Source: three-view drawing plus pictorial views. Frame: mm from the lowest corner of the part. Give positions to 0.01 mm unless a question says otherwise; leave off trailing zeros. Loops run counter-clockwise (first coordinate to the right, second up) from the corner with the lowest first, then second, coordinate; pieces in that order, holes last. Notation, with made-up numbers: (-37.75, 19.25) -> (-12.75, 19.25) arc R30 ccw to (-12.75, 52.25) -> close; hole circle Ø9 at (61, 20). An arc over 180 degrees is marked (long way). Put each result on its own line as item: value.
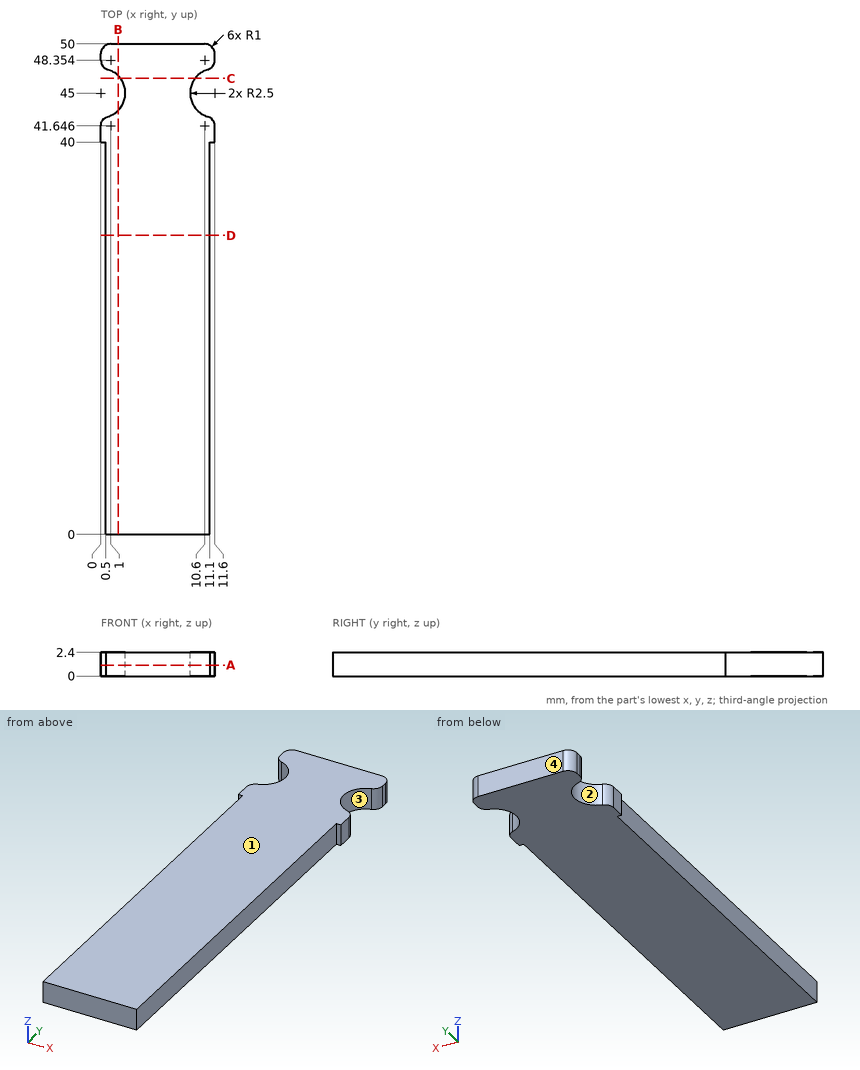
(1) Section C-C on y = 46.5. Return loops of the section in (x, z).
Calculated:
outline: (2, 0) -> (9.6, 0) -> (9.6, 2.4) -> (2, 2.4) -> close
(2) First-contact query: P1, Ø0.7, axis at y = 29, z = 1, coming from the -X side; P2, Ø0.6, axis at x = 11.5, z = 1, coming from the -Y side; P3, Ø0.7, axis at y = 30, z = 1.5, coming from the +X side. Flat tips, straight axial feed; report the tip coordinate or a pass-through.
Calculated:
P1: stops at x = 0.5
P2: stops at y = 40
P3: stops at x = 11.1
(3) Draft query along Y for the marked faces 1, 2, 3 and 4. Return one class per face: released by +Y, released by -Y, zero draft, split by the parting line, or undercut.
Calculated:
face 1: zero draft
face 2: undercut
face 3: undercut
face 4: released by +Y
(4) Section D-D on y = 30.5. Return loops of the section in (x, z), then the cut area to 3 significant figures.
Calculated:
outline: (0.5, 0) -> (11.1, 0) -> (11.1, 2.4) -> (0.5, 2.4) -> close
area: 25.4 mm²
(5) Line query: probe 1 along X at (y, z) = (7.5, 1.7); probe 2 along Y at (x, z) = (2, 0.8); probe 3 along Y at (x, z) = (1, 1.7). Output: solid intervals per line, ascending. Write a range as from..to.
Calculated:
probe 1: x = 0.5..11.1
probe 2: y = 0..43.5, 46.5..50
probe 3: y = 0..42.71, 47.29..50
(6) Section A-A on z = 1.1. Return loops of the section in (x, y).
Calculated:
outline: (0, 40) -> (0.5, 40) -> (0.5, 0) -> (11.1, 0) -> (11.1, 40) -> (11.6, 40) -> (11.6, 41.65) arc R1 ccw to (10.89, 42.6) arc R2.5 cw to (10.89, 47.4) arc R1 ccw to (11.6, 48.35) -> (11.6, 49) arc R1 ccw to (10.6, 50) -> (1, 50) arc R1 ccw to (0, 49) -> (0, 48.35) arc R1 ccw to (0.71, 47.4) arc R2.5 cw to (0.71, 42.6) arc R1 ccw to (0, 41.65) -> close
(7) Section B-B on x = 1.75. Return loops of the section in (y, z).
Calculated:
outline: (0, 0) -> (43.21, 0) -> (43.21, 2.4) -> (0, 2.4) -> close; (46.79, 0) -> (50, 0) -> (50, 2.4) -> (46.79, 2.4) -> close
